Print and shaded views of the part. All mm, measured from the part's lowest x, y and z. A direction names the side the tool comes from. Coordinates: 2 decimals unless noted, no trailing zeros. Loops run counter-clockwise (first coordinate to the right, second up) from the corner with the lowest first, then second, coordinate; pieces in that order, holes last. Notation, with made-up numbers: M 26.5,89.25 L 38.5,89.25 A31 cw 38.5,115.25 Z; hole C -26,-15 d1. An arc over 180 degrees is marked long. One line per question, with ' | ' between items. Start each with the question number.
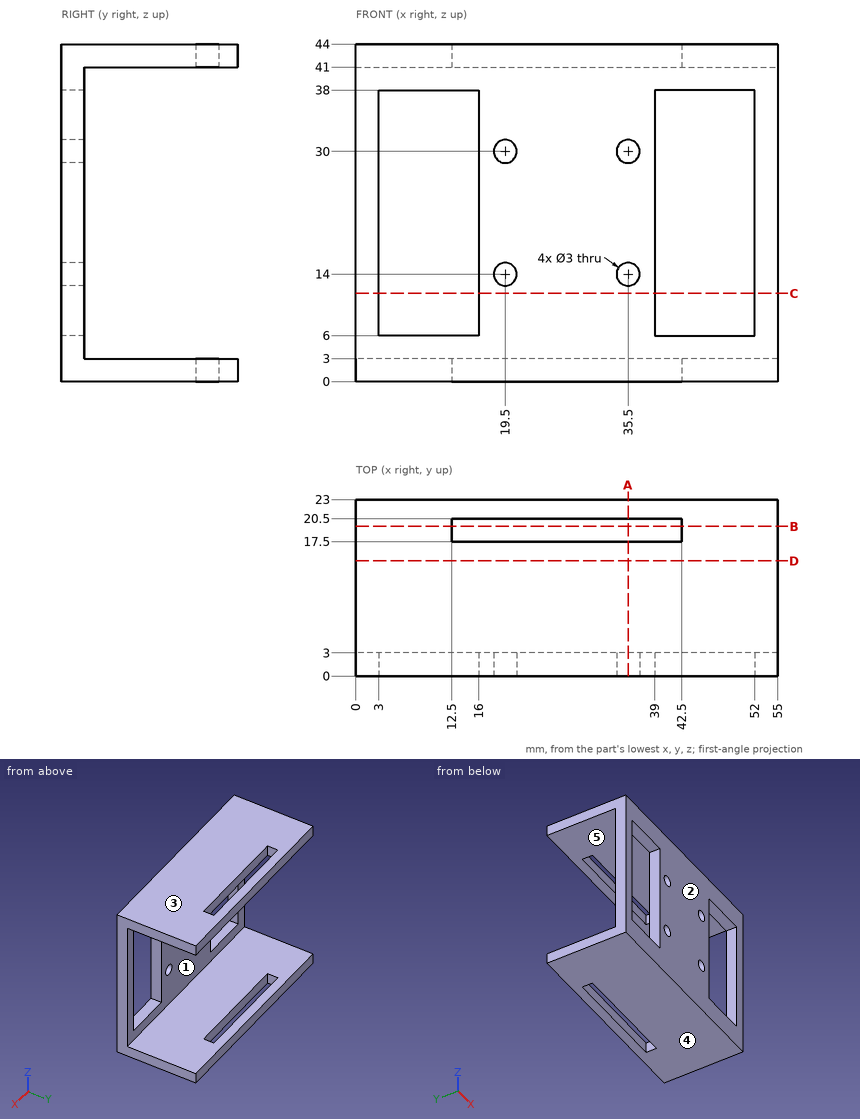
(1) Band-saw the part on B-B on y = 19.5. Write the cut outline in (x, z), then the cut area to 3 significant figures.
(2) Band-saw the part on A-A on x = 35.5. Write the cut outline in (y, z).
(3) Two-plate mould, pull along Z, no slides. Class the marked faces 1, 2 and 3: pulls with the +Z half, pulls with the -Z half, needs draft (parallel to the pull), parting line crosses it, or undercut.
(4) Pin check, flat tip, straight feed: P1, Ø5, axis at x = 35.5, z = 14, coming from the +Y side. Stop position of the tip, or through.
(5) Drill centre lines: line 1 (X direction, y = 2.1, z = 30); line 2 (Z direction, x = 35.5, y = 1.05); line 3 (Z direction, x = 52.5, y = 10.75). Where is each one in solid material? Low to high. Write a range as [from, to].
(6) Band-saw the part on D-D on y = 15. Write the cut outline in (x, z).
(7) 3-axis set-ups, long thin cutter, end or side, ignore diameter. For the marked faces 4 and 5: which of +Z, -Z, +X, -X, +Y, -Y reach the whole face in a straight line?
(8) Band-saw the part on C-C on z = 11.5. Write the cut outline in (x, y), then the cut area to 3 significant figures.
Computed values:
1) outline: M 0,0 L 12.5,0 L 12.5,3 L 0,3 Z; M 0,41 L 12.5,41 L 12.5,44 L 0,44 Z; M 42.5,0 L 55,0 L 55,3 L 42.5,3 Z; M 42.5,41 L 55,41 L 55,44 L 42.5,44 Z | area: 150 mm^2
2) outline: M 0,0 L 17.5,0 L 17.5,3 L 3,3 L 3,12.5 L 0,12.5 Z; M 0,15.5 L 3,15.5 L 3,28.5 L 0,28.5 Z; M 0,31.5 L 3,31.5 L 3,41 L 17.5,41 L 17.5,44 L 0,44 Z; M 20.5,0 L 23,0 L 23,3 L 20.5,3 Z; M 20.5,41 L 23,41 L 23,44 L 20.5,44 Z
3) face 1: undercut | face 2: needs draft | face 3: pulls with the +Z half
4) P1: y = 3
5) line 1: [0, 3], [16, 18], [21, 34], [37, 39], [52, 55] | line 2: [0, 12.5], [15.5, 28.5], [31.5, 44] | line 3: [0, 3], [41, 44]
6) outline: M 0,0 L 55,0 L 55,3 L 0,3 Z; M 0,41 L 55,41 L 55,44 L 0,44 Z
7) face 4: -Z, +X, -X, +Y, -Y | face 5: +X, -X, +Y
8) outline: M 0,0 L 3,0 L 3,3 L 0,3 Z; M 16,0 L 39,0 L 39,3 L 16,3 Z; M 52,0 L 55,0 L 55,3 L 52,3 Z | area: 87.0 mm^2
